from build123d import *

# Parameters (mm, degrees)
SKETCH1_W           = 92
SKETCH1_H           = 60
SKETCH1_R           = 4.05
SKETCH1_R_2         = 2.1
SKETCH1_R_3         = 2.5
BOSS_EXTRUDE1_DEPTH = 2.5
FILLET1_R           = 2


with BuildPart() as part:
    # Sketch1 → Boss-Extrude1 (new, symmetric)
    with BuildSketch(Plane.XY):
        Rectangle(SKETCH1_W, SKETCH1_H)
        Circle(SKETCH1_R, mode=Mode.SUBTRACT)
        with Locations((0, 17.5)):
            Circle(SKETCH1_R_2, mode=Mode.SUBTRACT)
        with Locations((0, -17.5)):
            Circle(SKETCH1_R_2, mode=Mode.SUBTRACT)
        with Locations((-17.5, 0)):
            Circle(SKETCH1_R_2, mode=Mode.SUBTRACT)
        with Locations((17.5, 0)):
            Circle(SKETCH1_R_2, mode=Mode.SUBTRACT)
        with Locations((29, 21.5)):
            Circle(SKETCH1_R_3, mode=Mode.SUBTRACT)
        with Locations((29, -21.5)):
            Circle(SKETCH1_R_3, mode=Mode.SUBTRACT)
        with Locations((-29, -21.5)):
            Circle(SKETCH1_R_3, mode=Mode.SUBTRACT)
        with Locations((-29, 21.5)):
            Circle(SKETCH1_R_3, mode=Mode.SUBTRACT)
        with Locations((-31, 0)):
            Circle(SKETCH1_R_2, mode=Mode.SUBTRACT)
        with Locations((31, 0)):
            Circle(SKETCH1_R_2, mode=Mode.SUBTRACT)
        with Locations((9.941037343, -25)):
            Circle(SKETCH1_R_2, mode=Mode.SUBTRACT)
        with Locations((-9.466357856, 25.166900153)):
            Circle(SKETCH1_R_2, mode=Mode.SUBTRACT)
        with BuildLine():
            Line((37.7, 20.5), (37.7, 22.5))
            ThreePointArc((37.7, 22.5), (39, 23.8), (40.3, 22.5))
            Line((40.3, 22.5), (40.3, 20.5))
            ThreePointArc((40.3, 20.5), (39, 19.2), (37.7, 20.5))
        make_face(mode=Mode.SUBTRACT)
        with BuildLine():
            Line((21.7, 20.5), (21.7, 22.5))
            ThreePointArc((21.7, 22.5), (23, 23.8), (24.3, 22.5))
            Line((24.3, 22.5), (24.3, 20.5))
            ThreePointArc((24.3, 20.5), (23, 19.2), (21.7, 20.5))
        make_face(mode=Mode.SUBTRACT)
        with BuildLine():
            Line((37.7, -20.5), (37.7, -22.5))
            ThreePointArc((37.7, -22.5), (39, -23.8), (40.3, -22.5))
            Line((40.3, -22.5), (40.3, -20.5))
            ThreePointArc((40.3, -20.5), (39, -19.2), (37.7, -20.5))
        make_face(mode=Mode.SUBTRACT)
        with BuildLine():
            Line((21.7, -20.5), (21.7, -22.5))
            ThreePointArc((21.7, -22.5), (23, -23.8), (24.3, -22.5))
            Line((24.3, -22.5), (24.3, -20.5))
            ThreePointArc((24.3, -20.5), (23, -19.2), (21.7, -20.5))
        make_face(mode=Mode.SUBTRACT)
        with BuildLine():
            Line((-21.7, -20.5), (-21.7, -22.5))
            ThreePointArc((-21.7, -22.5), (-23, -23.8), (-24.3, -22.5))
            Line((-24.3, -22.5), (-24.3, -20.5))
            ThreePointArc((-24.3, -20.5), (-23, -19.2), (-21.7, -20.5))
        make_face(mode=Mode.SUBTRACT)
        with BuildLine():
            Line((-37.7, -20.5), (-37.7, -22.5))
            ThreePointArc((-37.7, -22.5), (-39, -23.8), (-40.3, -22.5))
            Line((-40.3, -22.5), (-40.3, -20.5))
            ThreePointArc((-40.3, -20.5), (-39, -19.2), (-37.7, -20.5))
        make_face(mode=Mode.SUBTRACT)
        with BuildLine():
            Line((-21.7, 20.5), (-21.7, 22.5))
            ThreePointArc((-21.7, 22.5), (-23, 23.8), (-24.3, 22.5))
            Line((-24.3, 22.5), (-24.3, 20.5))
            ThreePointArc((-24.3, 20.5), (-23, 19.2), (-21.7, 20.5))
        make_face(mode=Mode.SUBTRACT)
        with BuildLine():
            Line((-37.7, 20.5), (-37.7, 22.5))
            ThreePointArc((-37.7, 22.5), (-39, 23.8), (-40.3, 22.5))
            Line((-40.3, 22.5), (-40.3, 20.5))
            ThreePointArc((-40.3, 20.5), (-39, 19.2), (-37.7, 20.5))
        make_face(mode=Mode.SUBTRACT)
    extrude(amount=BOSS_EXTRUDE1_DEPTH, both=True)

    # Fillet1
    fillet1_edges = [part.edges().sort_by_distance(p)[0] for p in [
        (-46, -30, 0),
        (-46, 30, 0),
        (46, 30, 0),
        (46, -30, 0),
    ]]
    fillet(fillet1_edges, radius=FILLET1_R)


solid = part.part
Verification items for the finished model (mm, model axes). A direction names the side the tool comes from. Round coordinates to 2 decimals unless told otherwise and drop trailing zeros. Loops run counter-clockwise (first coordinate to the right, second up) from the corner with the lowest first, then second, coordinate; pieces in that order, holes last. Notation, with made-up numbers: (58, 0.5) - (69, 0.5) arc R33 ccw to (69, 35.5) - close; hole circle Ø2 at (65, -20). An arc over 180 degrees is marked (long way). Use a Markdown table: item, result. Add a question column.
1. Thickness scan on probe 1 along Y at (x, z) = (0, 1.45); probe 2 along Y at (x, z) = (17.5, -1.05); probe 3 along Y at (x, z) = (-32, 1.15). Record the ranges inside material, lowest first. Write a range as [from, to].
2. Section check B-B, the plane y = 21.5. Record the boundary of the cut face in (x, z), plus the area to 3 significant figures.
3. Access from +Z, -Z, +X, -X, +Y, -Y to the whole of each face (thin tool, end or side, straight path). Record for faces 1 (the face through (23, 23.8, 0)), 2 (the face through (-1, 30, 0)).
4. Section check D-D, the plane y = -17.5. Record the boundary of the cut face in (x, z).
5. Release check for a two-part mould opening along X. For faces 3 (the face through (-1, 7, -2.5)), 4 (the face through (29, -19, 0)), 5 (the face through (-39, 19.2, 0)) record: released by +X, released by -X, zero draft, split by the parting line, or undercut.
6. Section check A-A, the plane x = -17.5. Record the boundary of the cut face in (y, z).
7. Section check C-C, the plane x = 27.5. Record the boundary of the cut face in (y, z), plus the area to 3 significant figures.
8. Gauge pin test, flat end, axial feed: pin 1 (5 mm diameter, centred on x = 0, y = 0, fed in from +Z). Record the tip position at first contact, or that the pin passes through.
Checks:
| question | item | result |
|---|---|---|
| 1 | probe 1 | y = [-30, -19.6], [-15.4, -4.05], [4.05, 15.4], [19.6, 30] |
| 1 | probe 2 | y = [-30, -2.1], [2.1, 30] |
| 1 | probe 3 | y = [-30, -1.85], [1.85, 30] |
| 2 | outline | (-46, -2.5) - (-40.3, -2.5) - (-40.3, 2.5) - (-46, 2.5) - close; (-37.7, -2.5) - (-31.5, -2.5) - (-31.5, 2.5) - (-37.7, 2.5) - close; (-26.5, -2.5) - (-24.3, -2.5) - (-24.3, 2.5) - (-26.5, 2.5) - close; (-21.7, -2.5) - (21.7, -2.5) - (21.7, 2.5) - (-21.7, 2.5) - close; (24.3, -2.5) - (26.5, -2.5) - (26.5, 2.5) - (24.3, 2.5) - close; (31.5, -2.5) - (37.7, -2.5) - (37.7, 2.5) - (31.5, 2.5) - close; (40.3, -2.5) - (46, -2.5) - (46, 2.5) - (40.3, 2.5) - close |
| 2 | area | 358 mm^2 |
| 3 | face 1 | +Z, -Z |
| 3 | face 2 | +Z, -Z, +X, -X, +Y |
| 4 | outline | (-46, -2.5) - (-2.1, -2.5) - (-2.1, 2.5) - (-46, 2.5) - close; (2.1, -2.5) - (46, -2.5) - (46, 2.5) - (2.1, 2.5) - close |
| 5 | face 3 | zero draft |
| 5 | face 4 | undercut |
| 5 | face 5 | undercut |
| 6 | outline | (-30, -2.5) - (-2.1, -2.5) - (-2.1, 2.5) - (-30, 2.5) - close; (2.1, -2.5) - (30, -2.5) - (30, 2.5) - (2.1, 2.5) - close |
| 7 | outline | (-30, -2.5) - (-23.5, -2.5) - (-23.5, 2.5) - (-30, 2.5) - close; (-19.5, -2.5) - (19.5, -2.5) - (19.5, 2.5) - (-19.5, 2.5) - close; (23.5, -2.5) - (30, -2.5) - (30, 2.5) - (23.5, 2.5) - close |
| 7 | area | 260 mm^2 |
| 8 | pin 1 | passes through |
